```python
from build123d import *

# Parameters (mm, degrees)
SKETCH_1_R          = 18
EXTRUDE_1_DEPTH     = 92
CUT_EXTRUDE_2_DEPTH = 36
SHELL_8_T           = -1
SKETCH_2_R          = 11
EXTRUDE_2_DEPTH     = 2
SKETCH_3_R          = 4
EXTRUDE_3_DEPTH     = 18
CUT_EXTRUDE_START   = -15
CUT_EXTRUDE_1_DEPTH = 15
SKETCH_5_R          = 5
EXTRUDE_4_DEPTH     = 3
SKETCH_6_R          = 1.5
EXTRUDE_5_DEPTH     = 1
FILLET_1_R          = 1
SKETCH_8_R          = 1.5
CUT_EXTRUDE_3_DEPTH = 5
SKETCH_9_W          = 0.3
SKETCH_9_H          = 9
SKETCH_9_H_2        = 5


with BuildPart() as part:
    # 草图1 → 凸台-拉伸1 (new body)
    with BuildSketch(Plane.XY):
        Circle(SKETCH_1_R)
    extrude(amount=EXTRUDE_1_DEPTH)

    # 草图7 → 切除-拉伸2 (cut)
    with BuildSketch(Plane(origin=(0, 18, 0), x_dir=(1, 0, 0), z_dir=(0, 1, 0))):
        with BuildLine():
            Line((5, -18), (-5, -18))
            ThreePointArc((-5, -18), (-8, -15), (-5, -12))
            Line((-5, -12), (5, -12))
            ThreePointArc((5, -12), (8, -15), (5, -18))
        make_face()
    extrude(amount=-CUT_EXTRUDE_2_DEPTH, mode=Mode.SUBTRACT)

    # 抽壳8
    shell_8_openings = [part.faces().sort_by_distance(p)[0] for p in [
        (8, 0, 15),
        (0, 0, 18),
        (-8, 0, 15),
        (0, 0, 12),
    ]]
    offset(amount=SHELL_8_T, openings=shell_8_openings)

    # 草图2 → 凸台-拉伸2 (add)
    with BuildSketch(Plane.XY.offset(92)):
        Circle(SKETCH_2_R)
    extrude(amount=EXTRUDE_2_DEPTH)

    # 草图3 → 凸台-拉伸3 (add)
    with BuildSketch(Plane.XY.offset(94)):
        Circle(SKETCH_3_R)
    extrude(amount=EXTRUDE_3_DEPTH)

    # 草图4 → 切除-拉伸1 (cut)
    with BuildSketch(Plane.XY.offset(112).offset(CUT_EXTRUDE_START)):
        with BuildLine():
            ThreePointArc((2.645751311, 3), (1.414213562, 3.741657387), (0, 4))
            Line((0, 4), (0, 3))
            Line((0, 3), (2.645751311, 3))
        make_face()
        with BuildLine():
            Line((0, 3), (0, 4))
            ThreePointArc((0, 4), (-1.414213562, 3.741657387), (-2.645751311, 3))
            Line((-2.645751311, 3), (0, 3))
        make_face()
    extrude(amount=CUT_EXTRUDE_1_DEPTH, mode=Mode.SUBTRACT)

    # 草图5 → 凸台-拉伸4 (add)
    with BuildSketch(Plane(origin=(0, 0, 0), x_dir=(-1, 0, 0), z_dir=(0, 0, -1))):
        with Locations(Location((0, 0, 0), (0, 0, 180))):
            Circle(SKETCH_5_R)
    extrude(amount=EXTRUDE_4_DEPTH)

    # 草图6 → 凸台-拉伸5 (add)
    with BuildSketch(Plane(origin=(0, 0, -3), x_dir=(-1, 0, 0), z_dir=(0, 0, -1))):
        Circle(SKETCH_6_R)
    extrude(amount=EXTRUDE_5_DEPTH)

    # 圆角1
    fillet_1_edges = [part.edges().sort_by_distance(p)[0] for p in [
        (-5, 0, -3),
        (1.5, 0, -4),
    ]]
    fillet(fillet_1_edges, radius=FILLET_1_R - 0.0001)  # a hair under: the kernel refuses the full size

    # 草图8 → 切除-拉伸3 (cut)
    with BuildSketch(Plane.XY.offset(92)):
        with Locations((14, 0)):
            Circle(SKETCH_8_R)
        with Locations((0, -14)):
            Circle(SKETCH_8_R)
        with Locations((-14, 0)):
            Circle(SKETCH_8_R)
        with Locations((0, 14)):
            Circle(SKETCH_8_R)
    extrude(amount=-CUT_EXTRUDE_3_DEPTH, mode=Mode.SUBTRACT)

    # 草图9 → 切除-旋转1 (revolve, cut)
    with BuildSketch(Plane(origin=(0, 0, 0), x_dir=(1, 0, 0), z_dir=(0, 1, 0)), mode=Mode.PRIVATE) as cut_revolve_1_sk:
        with Locations((17.85, -87.5)):
            Rectangle(SKETCH_9_W, SKETCH_9_H)
        with Locations((17.85, -61.5)):
            Rectangle(SKETCH_9_W, SKETCH_9_H_2)
    revolve(cut_revolve_1_sk.sketch.rotate(Axis((0, 0, 0), (0, 0, 1)), 180), axis=Axis((0, 0, 0), (0, 0, 1)), mode=Mode.SUBTRACT)


solid = part.part
```
Can you work these out from the model? Positions are in its coordinate system, mm. A direction names the side the tool comes from. Give positions to 0.01 mm unless a question says otherwise; leave off trailing zeros. Order: outer loops, then holes, each group sorted by start corner. A loop starts at its lowest first (then second) coordinate and runs counter-clockwise, first axis right, second up. Notation, with made-up numbers: (30, 9) - (57, 9) arc R23 ccw to (57, 29) - close; hole circle Ø5 at (82, 86). An arc over 180 degrees is marked (long way). Use a Markdown table: item, result. Add a question column.
Q1. If we section it at D-D on z = 98.5: Write out the boundary of the cut face in (x, y).
Q2. I'm going to push flat-ended pins straight in: pin 1 (4 mm diameter, centred on x = 11, z = 32, fed in from +Y); pin 2 (17.5 mm diameter, centred on x = 4, y = 4, fed in from +Z); pin 3 (12 mm diameter, centred on x = 1, y = -11.5, fed in from +Z); pin 4 (1.9 mm diameter, centred on x = 1.5, y = 17, fed in from +Z). Where does each tip first touch, or does it pass through?
Q3. If we mould it in two halves opening along Y, with no side actions, what happens to faces 1 (the cylindrical face through (12.5, 0.07, 91.51)), 2 (the flat face through (0, 3, 104)), 3 (the cylindrical face through (-5, 0, -1))? For each: released by +Y, released by -Y, zero draft, split by the parting line, or undercut.
Q4. If we section it at A-A on y = -9.5: Write out the boundary of the cut face in (x, z), plus the area to 3 significant figures.
Q5. Please list where these lines run through material, in increasing order: line 1 along Y through (x, z) = (0, 91.6); line 2 along Z through (x, y) = (4.5, 13.5); line 3 along Y through (x, z) = (0, 21).
Q6. If we section it at B-B on z = 26.5: Write out the boundary of the cut face in (x, y), plus the area to 3 significant figures.
Q7. On a 3-axis mill with a long thin cutter (end or side, diameter ignored), from which of +Z, -Z, +X, -X, +Y, -Y can I reach the whole of each face in a straight line? I mean faces 4 (the cylindrical face through (-2.213, 16.855, 45.37)), 5 (the cylindrical face through (-2.343, 17.847, 73.367)), 6 (the cylindrical face through (-0.325, 12.536, 91.507)), 7 (the cylindrical face through (-8, -15.9, 15.1)), 8 (the flat face through (4, -4, 0)). Say none if no direction works.
Q8. If we section it at C-C on x = -14: Write out the boundary of the cut face in (y, z).
Answers follow:
| question | item | result |
|---|---|---|
| 1 | outline | (-2.65, 3) arc R4 ccw (long way) to (2.65, 3) - close |
| 2 | pin 1 | stops at y = 15.59 |
| 2 | pin 2 | stops at z = 112 |
| 2 | pin 3 | stops at z = 94 |
| 2 | pin 4 | stops at z = 92 |
| 3 | face 1 | undercut |
| 3 | face 2 | released by +Y |
| 3 | face 3 | split by the parting line |
| 4 | outline | (-15.29, 0) - (15.29, 0) - (15.29, 59) - (14.93, 59) - (14.93, 64) - (15.29, 64) - (15.29, 83) - (14.93, 83) - (14.93, 92) - (5.55, 92) - (5.55, 94) - (-5.55, 94) - (-5.55, 92) - (-14.93, 92) - (-14.93, 83) - (-15.29, 83) - (-15.29, 64) - (-14.93, 64) - (-14.93, 59) - (-15.29, 59) - close; hole (-14.1, 1) - (14.1, 1) - (14.1, 91) - (-14.1, 91) - close |
| 4 | area | 288 mm^2 |
| 5 | line 1 | y = -17.7 to -15.5, -12.5 to 12.5, 15.5 to 17.7 |
| 5 | line 2 | z = 0 to 1, 91 to 92 |
| 5 | line 3 | y = -18 to -17, 17 to 18 |
| 6 | outline | circle Ø36 at (0, 0); hole circle Ø34 at (0, 0) |
| 6 | area | 110 mm^2 |
| 7 | face 4 | none |
| 7 | face 5 | +Z, -Z |
| 7 | face 6 | +Z |
| 7 | face 7 | +Y, -Y |
| 7 | face 8 | -Z |
| 8 | outline | (-11.31, 0) - (11.31, 0) - (11.31, 59) - (10.83, 59) - (10.83, 64) - (11.31, 64) - (11.31, 83) - (10.83, 83) - (10.83, 92) - (1.5, 92) - (1.5, 91) - (9.64, 91) - (9.64, 1) - (-9.64, 1) - (-9.64, 91) - (-1.5, 91) - (-1.5, 92) - (-10.83, 92) - (-10.83, 83) - (-11.31, 83) - (-11.31, 64) - (-10.83, 64) - (-10.83, 59) - (-11.31, 59) - close |
